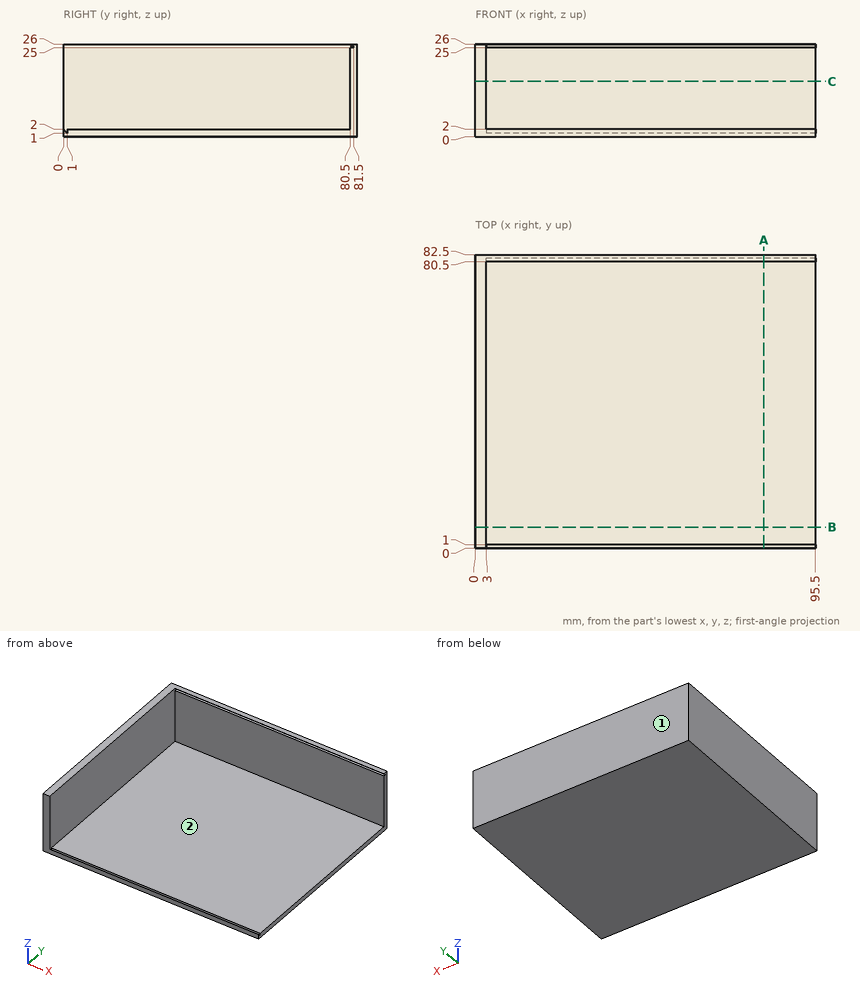
Answer from the drawing. Dimensions are ordinates in mm from the lowest x, y and z of the part. A direction names the side the tool comes from. Give positions to 0.01 mm unless a question says otherwise; leave off trailing zeros. Order: outer loops, then holes, each group sorted by start corner. A loop starts at its lowest first (then second) coordinate and runs counter-clockwise, first axis right, second up. Notation, with made-up numbers: (69.5, 64.5) -> (107.5, 64.5) arc R31 cw to (107.5, 97.5) -> close; hole circle Ø10 at (-34, -35.75). An arc over 180 degrees is marked (long way). One line per item, written item: value. Start each with the question number.
(1) A tool of negligible diameter and unlimited length cuts with its end or side. For the marked faces 1 and 2, from which of +Z, -Z, +X, -X, +Y, -Y can it reach the whole face along a straight path? Write none if from no direction.
(2) Straight lines are drawn through the part: L1, parallel to Y at x = 12.5, z = 19; L2, parallel to X at y = 68.5, z = 15; L3, parallel to Z at x = 46.5, y = 62. For each, find the intervals that lie inside material, in ascending order.
(3) The part is cut by section C-C (z = 15.5). Determine the outline of the cut face in (x, y).
(4) The part is cut by section A-A (x = 81). Determine the outline of the cut face in (y, z), and give its area (3 significant figures).
(5) The part is cut by section B-B (y = 6). Determine the outline of the cut face in (x, z), and give its area (3 significant figures).
(6) Flat-ended cylindrical pins translate along their axes: P1, Ø4, axis at y = 61.5, z = 15, coming from the +X side; P2, Ø3, axis at x = 83.5, y = 74, coming from the +Z side; P3, Ø2, axis at x = 66, z = 20, coming from the -Y side. Find the tip coordinate at first contact, or state that the pin passes through.
Taken from the geometry:
1. face 1: +Z, -Z, +X, -X, +Y
1. face 2: +Z, +X, -Y
2. L1: 80.5 to 82.5
2. L2: 0 to 3
2. L3: 0 to 2
3. outline: (0, 0) -> (3, 0) -> (3, 80.5) -> (95.5, 80.5) -> (95.5, 82.5) -> (0, 82.5) -> close
4. outline: (0, 0) -> (82.5, 0) -> (82.5, 26) -> (80.5, 26) -> (81.5, 25) -> (80.5, 25) -> (80.5, 2) -> (1, 2) -> (1, 1) -> (0, 2) -> close
4. area: 212 mm^2
5. outline: (0, 0) -> (95.5, 0) -> (95.5, 2) -> (3, 2) -> (3, 26) -> (0, 26) -> close
5. area: 263 mm^2
6. P1: x = 3
6. P2: z = 2
6. P3: y = 80.5
